from build123d import *

# Parameters (mm, degrees)
HEX_2_DEPTH = 2.3876


# Read off the part's stored shape, not the designer's step: ThreadSchematic
with BuildPart() as part:
    # ThreadSchematic outline → ThreadSchematic (revolve)
    with BuildSketch(Plane.YX):
        with BuildLine():
            Line((0, 23.8252), (0, 0))
            Line((0, 0), (3.9751, 0))
            Line((3.9751, 0), (4.7625, 0.7874))
            Line((4.7625, 0.7874), (4.7625, 4.7752))
            Line((4.7625, 4.7752), (3.1115, 4.7752))
            ThreePointArc((3.1115, 4.7752), (2.94985539, 4.84215539), (2.8829, 5.0038))
            Line((2.8829, 5.0038), (2.8829, 6.8707))
            Line((2.8829, 6.8707), (3.1496, 7.1374))
            Line((3.1496, 7.1374), (3.1496, 14.3002))
            Line((3.1496, 14.3002), (2.2733, 14.3002))
            ThreePointArc((2.2733, 14.3002), (1.860208218, 14.471308218), (1.6891, 14.8844))
            Line((1.6891, 14.8844), (1.6891, 16.4084))
            Line((1.6891, 16.4084), (2.413, 17.1323))
            Line((2.413, 17.1323), (2.413, 23.19528))
            Line((2.413, 23.19528), (1.78308, 23.8252))
            Line((1.78308, 23.8252), (0, 23.8252))
        make_face()
    revolve(axis=Axis((0, 0, 0), (1, 0, 0)))

    # Sketch2 → PreBroach (revolve, cut)
    with BuildSketch(Plane.XY, mode=Mode.PRIVATE) as prebroach_sk:
        Polygon((0, 1.5875), (2.3876, 1.5875), (3.304143552, 0), (0, 0), align=None)
    revolve(prebroach_sk.sketch.rotate(Axis((0, 0, 0), (1, 0, 0)), 90), axis=Axis((0, 0, 0), (1, 0, 0)), mode=Mode.SUBTRACT)

    # Sketch3 → Hex 2 (cut)
    with BuildSketch(Plane.ZY):
        Polygon((-1.5875, -0.916543552), (-1.5875, 0.916543552), (0, 1.833087105), (1.5875, 0.916543552), (1.5875, -0.916543552), (0, -1.833087105), align=None)
    extrude(amount=-HEX_2_DEPTH, mode=Mode.SUBTRACT)


solid = part.part
Here's how the part is built. I have some questions about the finished solid (model axes, mm). A direction names the side the tool comes from. Round coordinates to 2 decimals unless told otherwise and drop trailing zeros. Write each loop counter-clockwise with the first axis right and the second up, starting at its lowest first coordinate (ties: lowest second). Pieces come first, ordered by that corner, then holes.
1. For faces 4 (the flat face through (0, 0, -2)), 5 (the flat face through (14.3, 2, 2)), 6 (the cylindrical face through (10.769, -2.499, -1.916)), 7 (the flat face through (1.177, -1.381, -0.783)), which set-ups out of +Z, -Z, +X, -X, +Y, -Y let a thin tool reach every point of the face, with its end or its side?
2. Will these pins go through, and if not, where does the flat tip stop? pin 1 Ø2 at (x, y) = (8.5, -2.5) entering from -Z; pin 2 Ø1.5 at (x, z) = (13.5, 1.5) entering from +Y; pin 3 Ø3 at (x, z) = (5, 2.5) entering from -Y.
3. Suppose I cut it at B-B (x = 8.5). List the corners of the cut face in (y, z) for me, and give its area (3 significant figures).
4. If we mould it in two halves opening along Z, with no side actions, what happens to faces 1 (the cylindrical face through (15.66, -1.34, -1.03)), 2 (the flat face through (23.825, 0, 0)), 3 (the flat face through (1.177, 1.381, 0.783))? For each: released by +Z, released by -Z, zero draft, split by the parting line, or undercut.
5. I need wall thicknesses on L1, parallel to X at y = -1, z = -3.25; L2, parallel to Y at x = 1, z = 0.5; L3, parallel to X at y = -2.5, z = 1.25. Which ranges of each line are inside material? Lowest first, please.
6. Suppose I cut it at A-A (x = 19.75). List the corners of the cut face in (y, z) for me, and give its area (3 significant figures).
Answer sheet:
1. face 4: +Z, -Z, -X, +Y, -Y
1. face 5: none
1. face 6: +X
1. face 7: -X
2. pin 1: stops at z = -2.77
2. pin 2: stops at y = 3.06
2. pin 3: stops at y = -4.65
3. outline: circle Ø6.3 at (0, 0)
3. area: 31.2 mm2
4. face 1: split by the parting line
4. face 2: zero draft
4. face 3: undercut
5. L1: x = 0 to 4.78
5. L2: y = -4.74 to -1.54, 1.54 to 4.74
5. L3: x = 0 to 14.3
6. outline: circle Ø4.83 at (0, 0)
6. area: 18.3 mm2
